from build123d import *

# Parameters (mm, degrees)
SKETCH2_R                = 19.6
SKETCH2_R_2              = 12.25
BOSS_EXTRUDE1_DEPTH      = 22
BOSS_EXTRUDE2_DEPTH      = 55.75
BOSS_EXTRUDE2_DEPTH_BACK = 13
SKETCH3_R                = 17.25


with BuildPart() as part:
    # Sketch2 → Boss-Extrude1 (new body)
    with BuildSketch(Plane(origin=(0, 0, 0), x_dir=(1, 0, 0), z_dir=(0, 1, 0))):
        with Locations(Location((0, 0, 0), (0, 0, 270))):
            Circle(SKETCH2_R)
        with Locations(Location((0, 0, 0), (0, 0, 270))):
            Circle(SKETCH2_R_2, mode=Mode.SUBTRACT)
    extrude(amount=BOSS_EXTRUDE1_DEPTH)

    # Sketch3 → Boss-Extrude2 (add, two sides: drawn at the far end of the back side and taken through both)
    with BuildSketch(Plane(origin=(0, 22, 0), x_dir=(1, 0, 0), z_dir=(0, 1, 0)).offset(-BOSS_EXTRUDE2_DEPTH_BACK)):
        with Locations(Location((0, 0, 0), (0, 0, 270))):
            Circle(SKETCH3_R)
    extrude(amount=BOSS_EXTRUDE2_DEPTH + BOSS_EXTRUDE2_DEPTH_BACK)


solid = part.part
Build history of the part. All positions in model axes, mm. A direction names the side the tool comes from. Coordinates: 2 decimals unless noted, no trailing zeros. Write each loop counter-clockwise with the first axis right and the second up, starting at its lowest first coordinate (ties: lowest second). Pieces come first, ordered by that corner, then holes.
(1) Cut at D-D on z = 14. List the corners of the cut face in (x, y), and give its area (3 significant figures).
(2) Cut at B-B on x = 0. List the corners of the cut face in (y, z).
(3) Cut at A-A on z = 0. List the corners of the cut face in (x, y).
(4) 3-axis set-ups, long thin cutter, end or side, ignore diameter. For faces 4 (the flat face through (0, 9, 0)), 5 (the cylindrical face through (5.887, 10.846, 18.695)): which of +Z, -Z, +X, -X, +Y, -Y reach the whole face in a straight line?
(5) Drill centre lines: line 1 (X direction, y = 6, z = 0); line 2 (Y direction, x = 3.5, z = 10); line 3 (Y direction, x = -16, z = 9.5). Where is each one in solid material? Low to high.
(6) Mould opens along X. For faces 1 (the cylindrical face through (0.758, 49.485, -17.233)), 2 (the flat face through (-13, 22, 12)), 3 (the cylindrical face through (3.68, 4.437, 11.684)) say: pulls with the +X half, pulls with the -X half, needs draft (parallel to the pull), parting line crosses it, or undercut.
(7) Pin check, flat tips, straight feed: pin 1 Ø7.5 at (x, z) = (1.5, 2) entering from -Y; pin 2 Ø1.5 at (x, y) = (-8, 30) entering from +Z; pin 3 Ø1.5 at (y, z) = (35.5, -5) entering from +X. Stop position of each tip, or through.
(8) Cut at C-C on y = 71. List the corners of the cut face in (x, z), and give its area (3 significant figures).
Working result:
1. outline: (-13.72, 0) - (13.72, 0) - (13.72, 22) - (10.08, 22) - (10.08, 77.75) - (-10.08, 77.75) - (-10.08, 22) - (-13.72, 22) - close
1. area: 1,730 mm2
2. outline: (0, -19.6) - (22, -19.6) - (22, -17.25) - (77.75, -17.25) - (77.75, 17.25) - (22, 17.25) - (22, 19.6) - (0, 19.6) - (0, 12.25) - (9, 12.25) - (9, -12.25) - (0, -12.25) - close
3. outline: (-19.6, 0) - (-12.25, 0) - (-12.25, 9) - (12.25, 9) - (12.25, 0) - (19.6, 0) - (19.6, 22) - (17.25, 22) - (17.25, 77.75) - (-17.25, 77.75) - (-17.25, 22) - (-19.6, 22) - close
4. face 4: -Y
4. face 5: +Y, -Y
5. line 1: x = -19.6 to -12.25, 12.25 to 19.6
5. line 2: y = 9 to 77.75
5. line 3: y = 0 to 22
6. face 1: parting line crosses it
6. face 2: needs draft
6. face 3: undercut
7. pin 1: stops at y = 9
7. pin 2: stops at z = 15.65
7. pin 3: stops at x = 16.72
8. outline: circle Ø34.5 at (0, 0)
8. area: 935 mm2
